```python
from build123d import *

# Parameters (mm, degrees)
BOSS_EXTRUDE1_DEPTH                             = 135
CSK_FOR_M3_FLAT_HEAD_MACHINE_SCREW1_D           = 3.4
CSK_FOR_M3_FLAT_HEAD_MACHINE_SCREW1_DEPTH       = 5
CSK_FOR_M3_FLAT_HEAD_MACHINE_SCREW1_CSINK_D     = 6.3
CSK_FOR_M3_FLAT_HEAD_MACHINE_SCREW1_CSINK_ANGLE = 90
CSK_FOR_M3_FLAT_HEAD_MACHINE_SCREW1_TIP         = 1.021463052
CSK_FOR_M3_FLAT_HEAD_MACHINE_SCREW2_D           = 3.4
CSK_FOR_M3_FLAT_HEAD_MACHINE_SCREW2_DEPTH       = 5
CSK_FOR_M3_FLAT_HEAD_MACHINE_SCREW2_CSINK_D     = 6.3
CSK_FOR_M3_FLAT_HEAD_MACHINE_SCREW2_CSINK_ANGLE = 90
CSK_FOR_M3_FLAT_HEAD_MACHINE_SCREW2_TIP         = 1.021463052
FILLET1_R                                       = 4
CUT_EXTRUDE1_DEPTH                              = 10
LPATTERN1_COUNT                                 = 13
LPATTERN1_PITCH                                 = 6
CUT_EXTRUDE2_DEPTH                              = 10
LPATTERN2_COUNT                                 = 7
LPATTERN2_PITCH                                 = 6


with BuildPart() as part:
    # Sketch1 → Boss-Extrude1 (new body)
    with BuildSketch(Plane.XY):
        with BuildLine():
            Line((0, 0), (-2, 0))
            Line((-2, 0), (-2, 44.2))
            ThreePointArc((-2, 44.2), (-1.472792206, 45.472792206), (-0.2, 46))
            Line((-0.2, 46), (290.2, 46))
            ThreePointArc((290.2, 46), (291.472792206, 45.472792206), (292, 44.2))
            Line((292, 44.2), (292, 0))
            Line((292, 0), (290, 0))
            Line((290, 0), (290, 43.5))
            ThreePointArc((290, 43.5), (289.853553391, 43.853553391), (289.5, 44))
            Line((289.5, 44), (0.5, 44))
            ThreePointArc((0.5, 44), (0.146446609, 43.853553391), (0, 43.5))
            Line((0, 43.5), (0, 0))
        make_face()
    extrude(amount=BOSS_EXTRUDE1_DEPTH)

    # CSK for M3 Flat Head Machine Screw1
    with Locations(Plane.ZY.offset(2)):
        with Locations((8.5, 35), (8.5, 15), (126.5, 35), (126.5, 15)):
            CounterSinkHole(CSK_FOR_M3_FLAT_HEAD_MACHINE_SCREW1_D / 2, CSK_FOR_M3_FLAT_HEAD_MACHINE_SCREW1_CSINK_D / 2, depth=CSK_FOR_M3_FLAT_HEAD_MACHINE_SCREW1_DEPTH, counter_sink_angle=CSK_FOR_M3_FLAT_HEAD_MACHINE_SCREW1_CSINK_ANGLE)
            with Locations((0, 0, -(CSK_FOR_M3_FLAT_HEAD_MACHINE_SCREW1_DEPTH + CSK_FOR_M3_FLAT_HEAD_MACHINE_SCREW1_TIP / 2))):  # 118° drill point
                Cone(0, CSK_FOR_M3_FLAT_HEAD_MACHINE_SCREW1_D / 2, CSK_FOR_M3_FLAT_HEAD_MACHINE_SCREW1_TIP, mode=Mode.SUBTRACT)

    # CSK for M3 Flat Head Machine Screw2
    with Locations(Plane(origin=(292, 0, 0), x_dir=(0, 0, -1), z_dir=(1, 0, 0))):
        with Locations((-126.5, 35), (-126.5, 15), (-8.5, 35), (-8.5, 15)):
            CounterSinkHole(CSK_FOR_M3_FLAT_HEAD_MACHINE_SCREW2_D / 2, CSK_FOR_M3_FLAT_HEAD_MACHINE_SCREW2_CSINK_D / 2, depth=CSK_FOR_M3_FLAT_HEAD_MACHINE_SCREW2_DEPTH, counter_sink_angle=CSK_FOR_M3_FLAT_HEAD_MACHINE_SCREW2_CSINK_ANGLE)
            with Locations((0, 0, -(CSK_FOR_M3_FLAT_HEAD_MACHINE_SCREW2_DEPTH + CSK_FOR_M3_FLAT_HEAD_MACHINE_SCREW2_TIP / 2))):  # 118° drill point
                Cone(0, CSK_FOR_M3_FLAT_HEAD_MACHINE_SCREW2_D / 2, CSK_FOR_M3_FLAT_HEAD_MACHINE_SCREW2_TIP, mode=Mode.SUBTRACT)

    # Fillet1
    fillet1_edges = [part.edges().sort_by_distance(p)[0] for p in [
        (-1, 0, 0),
        (291, 0, 0),
        (291, 0, 135),
        (-1, 0, 135),
    ]]
    fillet(fillet1_edges, radius=FILLET1_R)

    # Sketch6 → Cut-Extrude1 (cut)
    with BuildSketch(Plane(origin=(-2, 0, 0), x_dir=(0, 0, -1), z_dir=(1, 0, 0))):
        with BuildLine():
            Line((-101.5, 38.35), (-101.5, 9.85))
            ThreePointArc((-101.5, 9.85), (-103.5, 7.85), (-105.5, 9.85))
            Line((-105.5, 9.85), (-105.5, 38.35))
            ThreePointArc((-105.5, 38.35), (-103.5, 40.35), (-101.5, 38.35))
        make_face()
    cut_extrude1 = extrude(amount=CUT_EXTRUDE1_DEPTH, mode=Mode.SUBTRACT)

    # LPattern1: Cut-Extrude1 ×13
    with Locations(*[(0, 0, -i * LPATTERN1_PITCH) for i in range(1, LPATTERN1_COUNT)]):
        add(cut_extrude1, mode=Mode.SUBTRACT)

    # Sketch7 → Cut-Extrude2 (cut)
    with BuildSketch(Plane(origin=(292, 0, 0), x_dir=(0, 0, -1), z_dir=(1, 0, 0))):
        with BuildLine():
            Line((-33.5, 38.35), (-33.5, 9.85))
            ThreePointArc((-33.5, 9.85), (-35.5, 7.85), (-37.5, 9.85))
            Line((-37.5, 9.85), (-37.5, 38.35))
            ThreePointArc((-37.5, 38.35), (-35.5, 40.35), (-33.5, 38.35))
        make_face()
    cut_extrude2 = extrude(amount=-CUT_EXTRUDE2_DEPTH, mode=Mode.SUBTRACT)

    # LPattern2: Cut-Extrude2 ×7
    with Locations(*[(0, 0, i * LPATTERN2_PITCH) for i in range(1, LPATTERN2_COUNT)]):
        add(cut_extrude2, mode=Mode.SUBTRACT)


solid = part.part
```
Verification items for the finished model (mm, model axes). A direction names the side the tool comes from. Coordinates: 2 decimals unless noted, no trailing zeros. Loops run counter-clockwise (first coordinate to the right, second up) from the corner with the lowest first, then second, coordinate; pieces in that order, holes last. Notation, with made-up numbers: (-21.5, 30) -> (26.5, 30) arc R25 cw to (26.5, 58) -> close; hole circle Ø9 at (77, -4). An arc over 180 degrees is marked (long way). Put each result on its own line as item: value.
1. Section check A-A, the plane y = 25. Give the number of separate pieces and of enclosed holes in the cut face, then the cut area to 3 significant figures.
Result set:
separate pieces: 22
enclosed holes: 0
area: 380 mm^2
2. Gauge pin test, flat ends, axial feed: P1, Ø3, axis at y = 37.5, z = 91.5, coming from the -X side; P2, Ø5.5, axis at y = 35, z = 8.5, coming from the -X side; P3, Ø3, axis at x = 67, z = 68.5, coming from the -Y side. Record the tip position at first contact, or that the pin passes through.
Result set:
P1: stops at x = 290
P2: stops at x = -1.6
P3: stops at y = 44
3. Thickness scan on line 1 (Y direction, x = 290.4, z = 126.5); line 2 (X direction, y = 43.5, z = 48.5); line 3 (Y direction, x = 208, z = 34). Record the ranges inside material, lowest first.
Result set:
line 1: y = 0 to 13.3, 16.7 to 33.3, 36.7 to 45.99
line 2: x = -2 to 0, 290 to 292
line 3: y = 44 to 46
4. Tool access check on faces 5 (the face through (147, 44, 67)), 6 (the face through (143, 46, 67)). Record the directions out of +Z, -Z, +X, -X, +Y, -Y that give a thin tool (end or side, any length) a straight path to the whole face; none if there is none.
Result set:
face 5: +Z, -Z, -Y
face 6: +Z, -Z, +X, -X, +Y
5. Mould release check, pull along X, two halves, no side actions. Record for faces 1 (the face through (146, 45, 135)), 2 (the face through (0, 7.6, 66.6)), 3 (the face through (292, 22, 82)), 4 (the face through (-2, 7, 67)): pulls with the +X half, pulls with the -X half, needs draft (parallel to the pull), parting line crosses it, or undercut.
Result set:
face 1: needs draft
face 2: undercut
face 3: pulls with the +X half
face 4: pulls with the -X half
6. Section check B-B, the plane x = 219.5. Record the boundary of the cut face in (y, z).
Result set:
outline: (44, 0) -> (46, 0) -> (46, 135) -> (44, 135) -> close
